```python
from build123d import *

# Parameters (mm, degrees)
SKETCH1_W            = 381
SKETCH1_H            = 207.9625
BOSS_EXTRUDE1_DEPTH  = 6.35
SKETCH2_W            = 25.4
SKETCH2_H            = 6.35
CUT_EXTRUDE1_DEPTH   = 6.35
LPATTERN1_COUNT      = 7
LPATTERN1_PITCH      = 50.8
SKETCH3_W            = 6.35
SKETCH3_H            = 41.5925
CUT_EXTRUDE2_DEPTH   = 6.35
LPATTERN2_COUNT      = 2
LPATTERN2_PITCH      = 83.185
SKETCH5_W            = 25.4
SKETCH5_H            = 6.35
CUT_EXTRUDE3_DEPTH   = 6.35
LPATTERN3_COUNT      = 7
LPATTERN3_PITCH      = 50.8
SKETCH6_W            = 6.35
SKETCH6_H            = 41.5925
CUT_EXTRUDE4_DEPTH   = 6.35
LPATTERN4_COUNT      = 2
LPATTERN4_PITCH      = 83.185
SKETCH7_R            = 1.778
CUT_EXTRUDE5_DEPTH   = 6.35
LPATTERN5_COUNT      = 13
LPATTERN5_PITCH      = 25.4
LPATTERN5_COUNT_DIR2 = 6
LPATTERN5_PITCH_DIR2 = 25.4


with BuildPart() as part:
    # Sketch1 → Boss-Extrude1 (new body)
    with BuildSketch(Plane.XY):
        Rectangle(SKETCH1_W, SKETCH1_H)
    extrude(amount=BOSS_EXTRUDE1_DEPTH)

    # Sketch2 → Cut-Extrude1 (cut)
    with BuildSketch(Plane.XY.offset(6.35)):
        with Locations((-152.4, 100.80625)):
            Rectangle(SKETCH2_W, SKETCH2_H)
    cut_extrude1 = extrude(amount=-CUT_EXTRUDE1_DEPTH, mode=Mode.SUBTRACT)

    # LPattern1: Cut-Extrude1 ×7
    with Locations(*[(i * LPATTERN1_PITCH, 0, 0) for i in range(1, LPATTERN1_COUNT)]):
        add(cut_extrude1, mode=Mode.SUBTRACT)

    # Sketch3 → Cut-Extrude2 (cut)
    with BuildSketch(Plane.XY.offset(6.35)):
        with Locations((-187.325, 41.5925)):
            Rectangle(SKETCH3_W, SKETCH3_H)
    cut_extrude2 = extrude(amount=-CUT_EXTRUDE2_DEPTH, mode=Mode.SUBTRACT)

    # LPattern2: Cut-Extrude2 ×2
    with Locations(*[(0, -i * LPATTERN2_PITCH, 0) for i in range(1, LPATTERN2_COUNT)]):
        add(cut_extrude2, mode=Mode.SUBTRACT)

    # Sketch5 → Cut-Extrude3 (cut)
    with BuildSketch(Plane.XY.offset(6.35)):
        with Locations((-152.4, -100.80625)):
            Rectangle(SKETCH5_W, SKETCH5_H)
    cut_extrude3 = extrude(amount=-CUT_EXTRUDE3_DEPTH, mode=Mode.SUBTRACT)

    # LPattern3: Cut-Extrude3 ×7
    with Locations(*[(i * LPATTERN3_PITCH, 0, 0) for i in range(1, LPATTERN3_COUNT)]):
        add(cut_extrude3, mode=Mode.SUBTRACT)

    # Sketch6 → Cut-Extrude4 (cut)
    with BuildSketch(Plane.XY.offset(6.35)):
        with Locations((187.325, 41.5925)):
            Rectangle(SKETCH6_W, SKETCH6_H)
    cut_extrude4 = extrude(amount=-CUT_EXTRUDE4_DEPTH, mode=Mode.SUBTRACT)

    # LPattern4: Cut-Extrude4 ×2
    with Locations(*[(0, -i * LPATTERN4_PITCH, 0) for i in range(1, LPATTERN4_COUNT)]):
        add(cut_extrude4, mode=Mode.SUBTRACT)

    # Sketch7 → Cut-Extrude5 (cut)
    with BuildSketch(Plane.XY.offset(6.35)):
        with Locations((-152.4, 65.88125)):
            Circle(SKETCH7_R)
    cut_extrude5 = extrude(amount=-CUT_EXTRUDE5_DEPTH, mode=Mode.SUBTRACT)

    # LPattern5: Cut-Extrude5 13 × 6
    with Locations(*[(i * LPATTERN5_PITCH, -j * LPATTERN5_PITCH_DIR2, 0) for i in range(LPATTERN5_COUNT) for j in range(LPATTERN5_COUNT_DIR2) if (i, j) != (0, 0)]):
        add(cut_extrude5, mode=Mode.SUBTRACT)


solid = part.part
```
Work out the finished part from the listing and answer in its coordinate system (mm). Give positions to 0.01 mm unless a question says otherwise; leave off trailing zeros. Loops run counter-clockwise (first coordinate to the right, second up) from the corner with the lowest first, then second, coordinate; pieces in that order, holes last. Notation, with made-up numbers: (-35.75, 46.25) - (-3.75, 46.25) arc R19 cw to (-3.75, 74.25) - close; hole circle Ø6 at (79, -25.5). An arc over 180 degrees is marked (long way). Use CSV: the item, a comma, the result in double quotes. Start each with the question number.
(1) Each of these flat-tipped pins is pushed along its axis until it touches: pin 1 (1 mm diameter, centred on y = -53.5, z = 4.5, fed in from -X); pin 2 (1.9 mm diameter, centred on x = -45, z = 2.5, fed in from +Y); pin 3 (1.9 mm diameter, centred on x = 52, z = 2.5, fed in from -Y); pin 4 (5.5 mm diameter, centred on x = 0, y = -35.72, fed in from -Z). Where does it stop, or does it pass through?
(2) Find the intervals of material crossed by L1, parallel to Y at x = -9, z = 1; L2, parallel to X at y = 28.5, z = 2.5, in increasing order.
(3) Find section B-B, the plane z = 2. Count the separate pieces of the cut face and the enclosed holes in it, plus the area to 3 significant figures.
(4) Find section C-C, the plane y = -44.5. Determine the outline of the cut face in (x, z).
(5) Find section A-A, the plane x = 60. Determine the outline of the cut face in (y, z).
Results found:
1,pin 1,"x = -184.15"
1,pin 2,"y = 97.63"
1,pin 3,"y = -97.63"
1,pin 4,"z = 0"
2,L1,"-97.63 to 97.63"
2,L2,"-184.15 to 184.15"
3,separate pieces,"1"
3,enclosed holes,"78"
3,area,"75,100 mm^2"
4,outline,"(-184.15, 0) - (184.15, 0) - (184.15, 6.35) - (-184.15, 6.35) - close"
5,outline,"(-97.63, 0) - (97.63, 0) - (97.63, 6.35) - (-97.63, 6.35) - close"
